Could you check a few things on this drawing? It's one solid part, dimensions in mm from its lowest x, y, z. A direction names the side the tool comes from. Coordinates: 2 decimals unless noted, no trailing zeros.
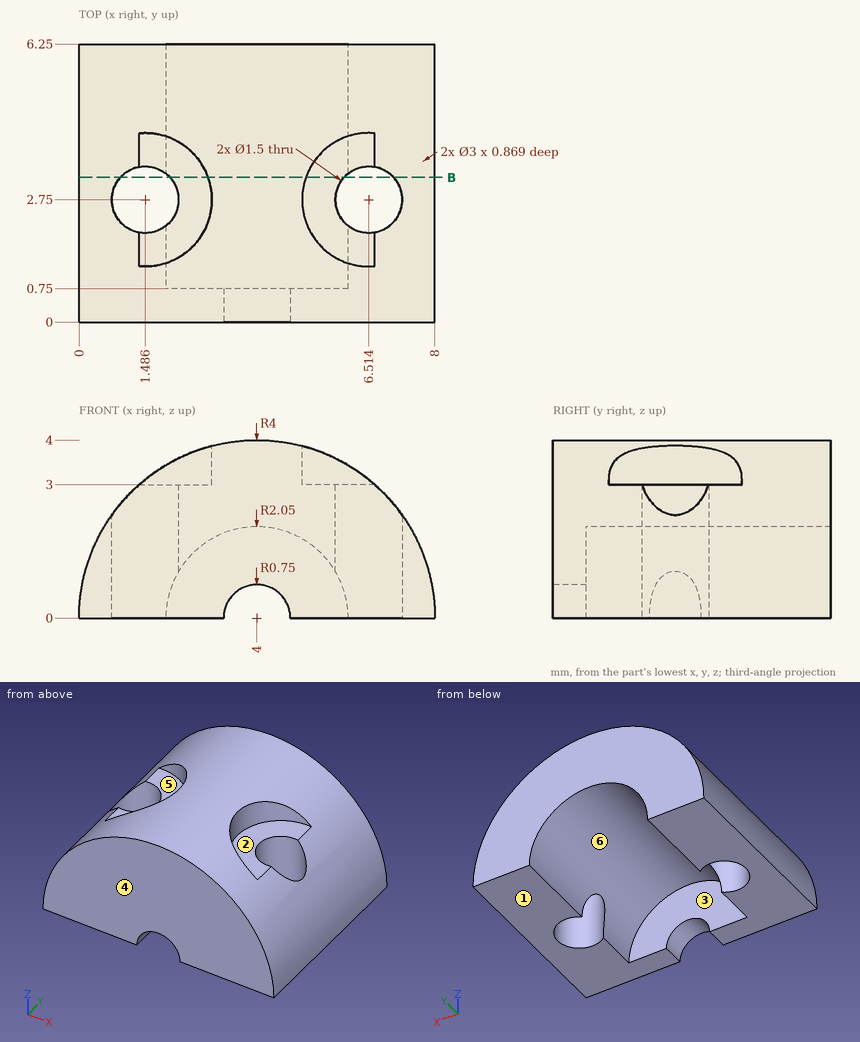
Q1. We'd pull the mould along Y, two halves only. Please class the marked faces 1, 2 and 3: pulls with the +Y half, pulls with the -Y half, needs draft (parallel to the pull), parting line crosses it, or undercut.
Q2. I need wall thicknesses on L1, parallel to Y at x = 1.5, z = 2.2; L2, parallel to X at y = 2.75, z = 3.6; L3, parallel to Z at x = 4, y = 4. Which ranges of each line are inside material? Lowest first, please.
Q3. If we section it at B-B on y = 3.25: Give the number of separate pieces and of enclosed holes in the cut face.
Q4. Will these pins go through, and if not, where does the flat tip stop? pin 1 (0.5 mm diameter, centred on x = 6, y = 2.5, fed in from +Z); pin 2 (1.7 mm diameter, centred on x = 6.51, y = 2.75, fed in from -Z); pin 3 (2 mm diameter, centred on x = 2.5, y = 1.5, fed in from +Z); pin 4 (1.8 mm diameter, centred on x = 2, y = 2, fed in from +Z) (1 decimal).
Q5. For the marked faces 4, 5 and 6, which set-ups out of +Z, -Z, +X, -X, +Y, -Y let a thin tool reach every point of the face, with its end or its side?
Reply:
1. face 1: needs draft
1. face 2: undercut
1. face 3: pulls with the +Y half
2. L1: y = 0 to 2, 3.5 to 6.25
2. L2: x = 2.99 to 5.01
2. L3: z = 2.05 to 4
3. separate pieces: 3
3. enclosed holes: 0
4. pin 1: stops at z = 3
4. pin 2: stops at z = 0
4. pin 3: stops at z = 3.97
4. pin 4: stops at z = 3.8
5. face 4: +Z, -Z, +X, -X, -Y
5. face 5: +Z, -X
5. face 6: -Z, +Y
